from build123d import *

# Parameters (mm, degrees)
FILLET1_R           = 1.5
FILLET2_R           = 0.5
FILLET3_R           = 1
FILLET4_R           = 0.5
SKETCH2_W           = 3
SKETCH2_H           = 1
BOSS_EXTRUDE1_DEPTH = 6


with BuildPart() as part:
    # Sketch1 → Revolve1 (revolve)
    with BuildSketch(Plane.XY, mode=Mode.PRIVATE) as revolve1_sk:
        with BuildLine():
            Line((6, 9), (6, 5.5))
            Line((6, 5.5), (9, 5.5))
            Line((9, 5.5), (9, 3.5))
            Line((9, 3.5), (7.5, 3.5))
            Line((7.5, 3.5), (7.5, -2.5))
            Line((7.5, -2.5), (6.5, -2.5))
            Line((6.5, -2.5), (6.5, -4.5))
            Line((6.5, -4.5), (5.5, -5))
            Line((5.5, -5), (5.5, -9))
            Line((5.5, -9), (0, -9))
            Line((0, -9), (0, 8.396096516))
            ThreePointArc((0, 8.396096516), (3.015157517, 8.547452829), (6, 9))
        make_face()
    revolve(revolve1_sk.sketch.rotate(Axis((0, -9, 0), (0, 1, 0)), 90), axis=Axis((0, -9, 0), (0, 1, 0)))

    # Fillet1
    fillet1_edges = [part.edges().sort_by_distance(p)[0] for p in [
        (0, 5.5, 9),
    ]]
    fillet(fillet1_edges, radius=FILLET1_R)

    # Fillet2
    fillet2_edges = [part.edges().sort_by_distance(p)[0] for p in [
        (0, 9, 6),
    ]]
    fillet(fillet2_edges, radius=FILLET2_R)

    # Fillet3
    fillet3_edges = [part.edges().sort_by_distance(p)[0] for p in [
        (0, -4.5, 6.5),
    ]]
    fillet(fillet3_edges, radius=FILLET3_R)

    # Fillet4
    fillet4_edges = [part.edges().sort_by_distance(p)[0] for p in [
        (0, -2.5, 7.5),
    ]]
    fillet(fillet4_edges, radius=FILLET4_R)

    # Sketch2 → Boss-Extrude1 (add)
    with BuildSketch(Plane.XZ.offset(9)):
        with Locations((0, 3)):
            Rectangle(SKETCH2_W, SKETCH2_H)
        with Locations((0, -3)):
            Rectangle(SKETCH2_W, SKETCH2_H)
    extrude(amount=BOSS_EXTRUDE1_DEPTH)


solid = part.part
CAD build for the part. Positions are in the model's coordinates, mm. A direction names the side the tool comes from. Coordinates: 2 decimals unless noted, no trailing zeros. Order: outer loops, then holes, each group sorted by start corner. A loop starts at its lowest first (then second) coordinate and runs counter-clockwise, first axis right, second up.
Item 1: Band-saw the part on C-C on y = -1.25. List the corners of the cut face in (x, z).
Check sheet entries:
outline: circle Ø15 at (0, 0)
Item 2: Band-saw the part on A-A on y = -11.75. List the corners of the cut face in (x, z).
Check sheet entries:
outline: (-1.5, -3.5) - (1.5, -3.5) - (1.5, -2.5) - (-1.5, -2.5) - close; (-1.5, 2.5) - (1.5, 2.5) - (1.5, 3.5) - (-1.5, 3.5) - close
Item 3: Band-saw the part on B-B on y = 6.25. List the corners of the cut face in (x, z), plus the area to 3 significant figures.
Check sheet entries:
outline: circle Ø12 at (0, 0)
area: 113 mm2
Item 4: Pin check, flat tips, straight feed: pin 1 Ø1.5 at (y, z) = (0, 6.5) entering from -X; pin 2 Ø0.8 at (y, z) = (-11, 3) entering from -X; pin 3 Ø10 at (y, z) = (-3, 4.5) entering from -X. Stop position of each tip, or through.
Check sheet entries:
pin 1: stops at x = -4.82
pin 2: stops at x = -1.5
pin 3: stops at x = -7.5
Item 5: Drill centre lines: L1, parallel to Z at x = -0.5, y = -9.25; L2, parallel to Z at x = -4.5, y = -1.75. Where is each one in solid material? Low to high.
Check sheet entries:
L1: z = -3.5 to -2.5, 2.5 to 3.5
L2: z = -6 to 6
Item 6: 3-axis set-ups, long thin cutter, end or side, ignore diameter. For faces 1 (the face through (-1.5, -12, 3)), 2 (the face through (-1.802, 6.927, -5.723)), 3 (the face through (1.5, -12, 3)), 4 (the face through (-4.393, -3.201, 4.791)): which of +Z, -Z, +X, -X, +Y, -Y reach the whole face in a straight line?
Check sheet entries:
face 1: +Z, -Z, -X, -Y
face 2: +Y
face 3: +Z, -Z, +X, -Y
face 4: -Y
